Design review of the part built by this model. Coordinates are the model's own, in mm. Face numbers are marked on the shaded views. A direction names the side the tool comes from. Coordinates: 2 decimals unless noted, no trailing zeros. Write each loop counter-clockwise with the first axis right and the second up, starting at its lowest first coordinate (ties: lowest second). Pieces come first, ordered by that corner, then holes. Notation, with made-up numbers: (45, 68) - (98, 68) arc R17 cw to (98, 97) - close; hole circle Ø4 at (70, 51). An arc over 180 degrees is marked (long way). Answer as CSV lines item,"result". Start each with the question number.
Q1. For line 1 along X through (y, z) = (-7, 9); line 2 along Z through (x, y) = (10.25, -120); line 3 along Z through (x, y) = (-7.5, -120), list the stretches that pass through material, from the lowest coordinate up. Write a range as [from, to].
Q2. Clearance check with flat-ended pins moving along their axes: pin 1 (4 mm diameter, centred on y = -30, z = 12, fed in from +X); pin 2 (4.5 mm diameter, centred on x = -1, y = -92, fed in from -Z). State where each tip first meets the part, or that it passes through.
Q3. Machinability: for the marked faces 1 and 2, which of the approach directions +Z, -Z, +X, -X, +Y, -Y give a long, thin tool a straight path to every point of the face, cutting with its end or side? Answer none if there is none.
Q4. We need section A-A (z = 12). Write out the cut boundary in (x, y).
Q5. We need section C-C (x = -2). Write out the cut boundary in (y, z).
Q6. Mouldability with a two-part tool opening along X and no side actions: class the marked faces 3, 4 and 5 as pulls with the +X half, pulls with the -X half, needs draft (parallel to the pull), parting line crosses it, or undercut.
Q7. We need section B-B (y = -120). Write out the cut boundary in (x, z).
from build123d import *

# Parameters (mm, degrees)
F1_DEPTH = 150
F2_R     = 3
F3_R     = 8
F4_R     = 2
F5_R     = 2.6
F6_DEPTH = 39


with BuildPart() as f1:
    # F0 (on Front) → F1 (new body)
    with BuildSketch(Plane.XZ):
        Polygon((-20.242574, 50), (-20.242574, 0), (-8.242574, 0), (-8.242574, 20), (6.757426, 20), (6.757426, 0), (18.757426, 0), (18.757426, 50), align=None)
    extrude(amount=F1_DEPTH)

    # F2
    f2_edges = [f1.edges().sort_by_distance(p)[0] for p in [
        (-8.242574, -75, 0),
        (6.757426, -75, 0),
    ]]
    fillet(f2_edges, radius=F2_R)

    # F3
    f3_edges = [f1.edges().sort_by_distance(p)[0] for p in [
        (-20.242574, -75, 50),
        (18.757426, -75, 50),
    ]]
    fillet(f3_edges, radius=F3_R)

    # F4
    f4_edges = [f1.edges().sort_by_distance(p)[0] for p in [
        (18.757426, -75, 0),
        (-20.242574, -75, 0),
    ]]
    fillet(f4_edges, radius=F4_R)

    # F5 (on face) → F6 (cut, through all)
    with BuildSketch(Plane(origin=(-20.242574, 0, 0), x_dir=(0, -1, 0), z_dir=(-1, 0, 0))):
        with Locations((30, 12)):
            Circle(F5_R)
        with Locations((120, 12)):
            Circle(F5_R)
    extrude(amount=-F6_DEPTH, mode=Mode.SUBTRACT)


solid = f1.part
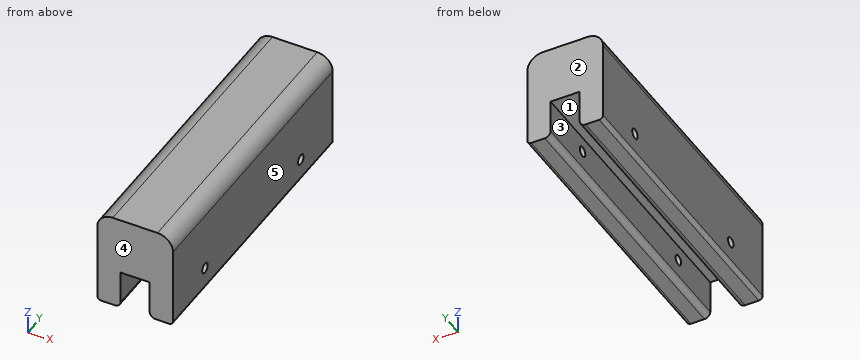
Results list:
1,line 1,"x = [-20.24, -8.24], [6.76, 18.76]"
1,line 2,"z = [0, 9.4], [14.6, 50]"
1,line 3,"z = [20, 50]"
2,pin 1,"passes through"
2,pin 2,"stops at z = 20"
3,face 1,"-Z, +Y, -Y"
3,face 2,"+Z, -Z, +X, -X, +Y"
4,outline,"(-20.24, -150) - (-8.24, -150) - (-8.24, -122.6) - (-20.24, -122.6) - close; (-20.24, -117.4) - (-8.24, -117.4) - (-8.24, -32.6) - (-20.24, -32.6) - close; (-20.24, -27.4) - (-8.24, -27.4) - (-8.24, 0) - (-20.24, 0) - close; (6.76, -150) - (18.76, -150) - (18.76, -122.6) - (6.76, -122.6) - close; (6.76, -117.4) - (18.76, -117.4) - (18.76, -32.6) - (6.76, -32.6) - close; (6.76, -27.4) - (18.76, -27.4) - (18.76, 0) - (6.76, 0) - close"
5,outline,"(-150, 20) - (0, 20) - (0, 50) - (-150, 50) - close"
6,face 3,"undercut"
6,face 4,"needs draft"
6,face 5,"pulls with the +X half"
7,outline,"(-20.24, 2) arc R2 ccw to (-18.24, 0) - (-11.24, 0) arc R3 ccw to (-8.24, 3) - (-8.24, 9.4) - (-20.24, 9.4) - close; (-20.24, 14.6) - (-8.24, 14.6) - (-8.24, 20) - (6.76, 20) - (6.76, 14.6) - (18.76, 14.6) - (18.76, 42) arc R8 ccw to (10.76, 50) - (-12.24, 50) arc R8 ccw to (-20.24, 42) - close; (6.76, 3) arc R3 ccw to (9.76, 0) - (16.76, 0) arc R2 ccw to (18.76, 2) - (18.76, 9.4) - (6.76, 9.4) - close"
